The listing builds one solid part. Answer for the finished solid, in the listing's coordinates (mm). A direction names the side the tool comes from. Give positions to 0.01 mm unless a question says otherwise; leave off trailing zeros. Order: outer loops, then holes, each group sorted by start corner. A loop starts at its lowest first (then second) coordinate and runs counter-clockwise, first axis right, second up. Notation, with made-up numbers: (-11.5, 2) - (-3.5, 2) arc R17 cw to (-3.5, 20) - close; hole circle Ø6 at (4.25, -36). An arc over 180 degrees is marked (long way). Answer in a Markdown table with one row per item.
from build123d import *

# Parameters (mm, degrees)
F0_W     = 39.6377146244
F0_H     = 78.2129243016
F1_DEPTH = 5
F2_W     = 39.6377146244
F2_H     = 4.4546872377
F3_DEPTH = 70
F4_W     = 39.6377146244
F4_H     = 8.1823468208
F5_DEPTH = 25
F7_DEPTH = 25


with BuildPart() as f1:
    # F0 (on Top) → F1 (new body)
    with BuildSketch(Plane.XY):
        with Locations((19.8188573122, 39.1064621508)):
            Rectangle(F0_W, F0_H)
    extrude(amount=F1_DEPTH)

    # F2 (on face) → F3 (join)
    with BuildSketch(Plane.XY.offset(5)):
        with Locations((19.8188573122, 75.9855806828)):
            Rectangle(F2_W, F2_H)
    extrude(amount=F3_DEPTH)

    # F4 (on face) → F5 (join)
    with BuildSketch(Plane.XY.offset(5)):
        with Locations((19.8188573122, 4.0911734104)):
            Rectangle(F4_W, F4_H)
    extrude(amount=F5_DEPTH)

    # F6 (on face) → F7 (cut)
    with BuildSketch(Plane.XZ):
        with BuildLine():
            ThreePointArc((0, 15), (19.8188573122, 29.9098357825), (39.6377146244, 15))
            Line((39.6377146244, 15), (39.6377146244, 30))
            Line((39.6377146244, 30), (0, 30))
            Line((0, 30), (0, 15))
        make_face()
    extrude(amount=-F7_DEPTH, mode=Mode.SUBTRACT)


solid = f1.part
Item 1: Find section D-D on z = 45.5. Write down the section's boundary in (x, y), then the cut area to 3 significant figures.
Answer block:
| item | result |
|---|---|
| outline | (0, 73.76) - (39.64, 73.76) - (39.64, 78.21) - (0, 78.21) - close |
| area | 177 mm² |
Item 2: Which of the six approach directions +Z, -Z, +X, -X, +Y, -Y give full straight-line access (tool end or side, diameter ignored) to faces 1 (the face through (19.446, 4.034, 29.906)), 2 (the face through (20, 8.182, 15)), 3 (the face through (20, 40, 0))?
Answer block:
| item | result |
|---|---|
| face 1 | +Z, -Y |
| face 2 | +Z, +X, -X |
| face 3 | -Z, +X, -X, +Y, -Y |
Item 3: Consider line 1 (Y direction, x = 25.5, z = 18.5); line 2 (Y direction, x = 23, z = 42); line 3 (Z direction, x = 14, y = 43). Determine where each line is inside the solid, lowest interval first.
Answer block:
| item | result |
|---|---|
| line 1 | 0 to 8.18, 73.76 to 78.21 |
| line 2 | 73.76 to 78.21 |
| line 3 | 0 to 5 |
Item 4: Find section B-B on x = 22.5. Write down the section's boundary in (y, z).
Answer block:
| item | result |
|---|---|
| outline | (0, 0) - (78.21, 0) - (78.21, 75) - (73.76, 75) - (73.76, 5) - (8.18, 5) - (8.18, 29.73) - (0, 29.73) - close |
Item 5: Find section C-C on y = 66. Write down the section's boundary in (x, z).
Answer block:
| item | result |
|---|---|
| outline | (0, 0) - (39.64, 0) - (39.64, 5) - (0, 5) - close |
Item 6: Each of these flat-tipped pins is pushed along its axis until it touches: P1, Ø10, axis at x = 17, y = 68.5, coming from the +Z side; P2, Ø8, axis at x = 22, z = 54.5, coming from the -Y side. Where does it stop, or does it pass through?
Answer block:
| item | result |
|---|---|
| P1 | z = 5 |
| P2 | y = 73.76 |
Item 7: Find section A-A on z = 10.5. Write down the section's boundary in (x, y), then the cut area to 3 significant figures.
Answer block:
| item | result |
|---|---|
| outline | (0, 0) - (39.64, 0) - (39.64, 8.18) - (0, 8.18) - close; (0, 73.76) - (39.64, 73.76) - (39.64, 78.21) - (0, 78.21) - close |
| area | 501 mm² |
